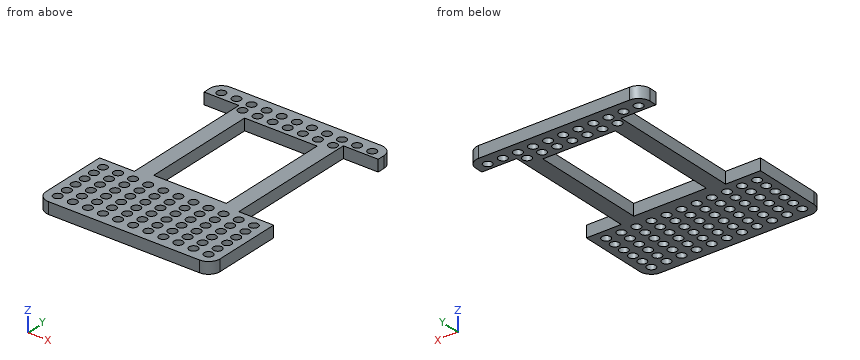
```python
from build123d import *

# Parameters (mm, degrees)
EXTRUDE_1_DEPTH     = 4
SKETCH_3_R          = 1.5
CUT_EXTRUDE_2_DEPTH = 4
SKETCH_5_W          = 12
SKETCH_5_H          = 46
CUT_EXTRUDE_3_DEPTH = 10
SKETCH_6_W          = 25
SKETCH_6_H          = 40
CUT_EXTRUDE_4_DEPTH = 10


with BuildPart() as part:
    # Эскиз1 → Бобышка-Вытянуть1 (new body)
    with BuildSketch(Plane.XY):
        with BuildLine():
            Line((4, 0), (56, 0))
            ThreePointArc((56, 0), (58.828427125, 1.171572875), (60, 4))
            Line((60, 4), (60, 76))
            ThreePointArc((60, 76), (58.828427125, 78.828427125), (56, 80))
            Line((56, 80), (4, 80))
            ThreePointArc((4, 80), (1.171572875, 78.828427125), (0, 76))
            Line((0, 76), (0, 4))
            ThreePointArc((0, 4), (1.171572875, 1.171572875), (4, 0))
        make_face()
    extrude(amount=EXTRUDE_1_DEPTH)

    # Эскиз3 → Вырез-Вытянуть2 (cut)
    with BuildSketch(Plane.XY.offset(4)):
        with Locations((4, 76)):
            Circle(SKETCH_3_R)
        with Locations((9.2, 76)):
            Circle(SKETCH_3_R)
        with Locations((14.4, 76)):
            Circle(SKETCH_3_R)
        with Locations((19.6, 76)):
            Circle(SKETCH_3_R)
        with Locations((24.8, 76)):
            Circle(SKETCH_3_R)
        with Locations((30, 76)):
            Circle(SKETCH_3_R)
        with Locations((35.2, 76)):
            Circle(SKETCH_3_R)
        with Locations((40.4, 76)):
            Circle(SKETCH_3_R)
        with Locations((45.6, 76)):
            Circle(SKETCH_3_R)
        with Locations((50.8, 76)):
            Circle(SKETCH_3_R)
        with Locations((56, 76)):
            Circle(SKETCH_3_R)
        with Locations((14.4, 72)):
            Circle(SKETCH_3_R)
        with Locations((19.6, 72)):
            Circle(SKETCH_3_R)
        with Locations((24.8, 72)):
            Circle(SKETCH_3_R)
        with Locations((30, 72)):
            Circle(SKETCH_3_R)
        with Locations((35.2, 72)):
            Circle(SKETCH_3_R)
        with Locations((40.4, 72)):
            Circle(SKETCH_3_R)
        with Locations((45.6, 72)):
            Circle(SKETCH_3_R)
        with Locations((14.4, 20)):
            Circle(SKETCH_3_R)
        with Locations((19.6, 20)):
            Circle(SKETCH_3_R)
        with Locations((24.8, 20)):
            Circle(SKETCH_3_R)
        with Locations((30, 20)):
            Circle(SKETCH_3_R)
        with Locations((35.2, 20)):
            Circle(SKETCH_3_R)
        with Locations((40.4, 20)):
            Circle(SKETCH_3_R)
        with Locations((45.6, 20)):
            Circle(SKETCH_3_R)
        with Locations((14.4, 16)):
            Circle(SKETCH_3_R)
        with Locations((19.6, 16)):
            Circle(SKETCH_3_R)
        with Locations((24.8, 16)):
            Circle(SKETCH_3_R)
        with Locations((30, 16)):
            Circle(SKETCH_3_R)
        with Locations((35.2, 16)):
            Circle(SKETCH_3_R)
        with Locations((40.4, 16)):
            Circle(SKETCH_3_R)
        with Locations((45.6, 16)):
            Circle(SKETCH_3_R)
        with Locations((14.4, 12)):
            Circle(SKETCH_3_R)
        with Locations((19.6, 12)):
            Circle(SKETCH_3_R)
        with Locations((24.8, 12)):
            Circle(SKETCH_3_R)
        with Locations((30, 12)):
            Circle(SKETCH_3_R)
        with Locations((35.2, 12)):
            Circle(SKETCH_3_R)
        with Locations((40.4, 12)):
            Circle(SKETCH_3_R)
        with Locations((45.6, 12)):
            Circle(SKETCH_3_R)
        with Locations((4, 8)):
            Circle(SKETCH_3_R)
        with Locations((9.2, 8)):
            Circle(SKETCH_3_R)
        with Locations((14.4, 8)):
            Circle(SKETCH_3_R)
        with Locations((19.6, 8)):
            Circle(SKETCH_3_R)
        with Locations((24.8, 8)):
            Circle(SKETCH_3_R)
        with Locations((30, 8)):
            Circle(SKETCH_3_R)
        with Locations((35.2, 8)):
            Circle(SKETCH_3_R)
        with Locations((40.4, 8)):
            Circle(SKETCH_3_R)
        with Locations((45.6, 8)):
            Circle(SKETCH_3_R)
        with Locations((50.8, 8)):
            Circle(SKETCH_3_R)
        with Locations((56, 8)):
            Circle(SKETCH_3_R)
        with Locations((4, 4)):
            Circle(SKETCH_3_R)
        with Locations((9.2, 4)):
            Circle(SKETCH_3_R)
        with Locations((14.4, 4)):
            Circle(SKETCH_3_R)
        with Locations((19.6, 4)):
            Circle(SKETCH_3_R)
        with Locations((24.8, 4)):
            Circle(SKETCH_3_R)
        with Locations((30, 4)):
            Circle(SKETCH_3_R)
        with Locations((35.2, 4)):
            Circle(SKETCH_3_R)
        with Locations((40.4, 4)):
            Circle(SKETCH_3_R)
        with Locations((45.6, 4)):
            Circle(SKETCH_3_R)
        with Locations((50.8, 4)):
            Circle(SKETCH_3_R)
        with Locations((56, 4)):
            Circle(SKETCH_3_R)
        with Locations((50.85, 20)):
            Circle(SKETCH_3_R)
        with Locations((50.85, 16)):
            Circle(SKETCH_3_R)
        with Locations((50.85, 12)):
            Circle(SKETCH_3_R)
        with Locations((56.1, 20)):
            Circle(SKETCH_3_R)
        with Locations((56.1, 16)):
            Circle(SKETCH_3_R)
        with Locations((56.1, 12)):
            Circle(SKETCH_3_R)
        with Locations((3.9, 20)):
            Circle(SKETCH_3_R)
        with Locations((3.9, 16)):
            Circle(SKETCH_3_R)
        with Locations((3.9, 12)):
            Circle(SKETCH_3_R)
        with Locations((9.15, 12)):
            Circle(SKETCH_3_R)
        with Locations((9.15, 16)):
            Circle(SKETCH_3_R)
        with Locations((9.15, 20)):
            Circle(SKETCH_3_R)
        with Locations((3.9, 24)):
            Circle(SKETCH_3_R)
        with Locations((9.1, 24)):
            Circle(SKETCH_3_R)
        with Locations((14.3, 24)):
            Circle(SKETCH_3_R)
        with Locations((19.5, 24)):
            Circle(SKETCH_3_R)
        with Locations((24.7, 24)):
            Circle(SKETCH_3_R)
        with Locations((29.9, 24)):
            Circle(SKETCH_3_R)
        with Locations((35.1, 24)):
            Circle(SKETCH_3_R)
        with Locations((40.3, 24)):
            Circle(SKETCH_3_R)
        with Locations((45.5, 24)):
            Circle(SKETCH_3_R)
        with Locations((50.7, 24)):
            Circle(SKETCH_3_R)
        with Locations((55.9, 24)):
            Circle(SKETCH_3_R)
    extrude(amount=-CUT_EXTRUDE_2_DEPTH, mode=Mode.SUBTRACT)

    # Эскиз5 → Вырез-Вытянуть3 (cut)
    with BuildSketch(Plane.XY.offset(4)):
        with Locations((6, 50.5)):
            Rectangle(SKETCH_5_W, SKETCH_5_H)
        with Locations((54, 50.5)):
            Rectangle(SKETCH_5_W, SKETCH_5_H)
    extrude(amount=-CUT_EXTRUDE_3_DEPTH, mode=Mode.SUBTRACT)

    # Эскиз6 → Вырез-Вытянуть4 (cut)
    with BuildSketch(Plane.XY.offset(4)):
        with Locations((30, 49)):
            Rectangle(SKETCH_6_W, SKETCH_6_H)
    extrude(amount=-CUT_EXTRUDE_4_DEPTH, mode=Mode.SUBTRACT)


solid = part.part
```
Geometry check sheet. Reference: the model listing, model coordinates, mm. Coordinates: 2 decimals unless noted, no trailing zeros. Loops run counter-clockwise (first coordinate to the right, second up) from the corner with the lowest first, then second, coordinate; pieces in that order, holes last.
Item 1: Sectioned sample at B-B, the plane z = 0.9. Count the separate pieces of the cut face and the enclosed holes in it, then the cut area to 3 significant figures.
Item 2: Sectioned sample at A-A, the plane y = 38. Record the boundary of the cut face in (x, z).
Item 3: Thickness scan on line 1 (Y direction, x = 38, z = 3.55); line 2 (X direction, y = 57, z = 1.25); line 3 (Y direction, x = 6, z = 1.8). Record the ranges inside material, lowest first.
Item 4: Go/stop test with flat-tipped pins: pin 1 Ø2.5 at (x, y) = (56, 76) entering from +Z; pin 2 Ø4 at (x, y) = (40.4, 72) entering from -Z. Record where each tip stops, or that it passes through.
Check result:
1. separate pieces: 1
1. enclosed holes: 85
1. area: 2,090 mm2
2. outline: (12, 0) - (17.5, 0) - (17.5, 4) - (12, 4) - close; (42.5, 0) - (48, 0) - (48, 4) - (42.5, 4) - close
3. line 1: y = 0 to 29, 69 to 80
3. line 2: x = 12 to 17.5, 42.5 to 48
3. line 3: y = 0 to 27.5, 73.5 to 80
4. pin 1: passes through
4. pin 2: stops at z = 0
